```python
from build123d import *
from OCP.BRepFilletAPI import BRepFilletAPI_MakeChamfer

# Parameters (mm, degrees)
SKETCH1_W           = 80
SKETCH1_H           = 60
BOSS_EXTRUDE2_DEPTH = 5
SKETCH3_W           = 15
SKETCH3_H           = 30
BOSS_EXTRUDE3_DEPTH = 25
SKETCH5_R           = 4.1
CUT_EXTRUDE2_DEPTH  = 105.403065089
CHAMFER1_SIZE       = 30
CHAMFER1_SIZE_2     = 10
FILLET1_R           = 15
SKETCH6_R           = 1.5
CUT_EXTRUDE3_DEPTH  = 105.403065089
SKETCH8_R           = 2.5
CUT_EXTRUDE5_DEPTH  = 104.07764064


with BuildPart() as part:
    # Sketch1 → Boss-Extrude2 (new body)
    with BuildSketch(Plane(origin=(0, 0, 0), x_dir=(1, 0, 0), z_dir=(0, 1, 0))):
        with Locations((40, 30)):
            Rectangle(SKETCH1_W, SKETCH1_H)
    extrude(amount=BOSS_EXTRUDE2_DEPTH)

    # Sketch3 → Boss-Extrude3 (add)
    with BuildSketch(Plane(origin=(0, 5, 0), x_dir=(1, 0, 0), z_dir=(0, 1, 0))):
        with Locations((72.5, 45)):
            Rectangle(SKETCH3_W, SKETCH3_H)
        with Locations((47.5, 45)):
            Rectangle(SKETCH3_W, SKETCH3_H)
        with Locations((22.5, 45)):
            Rectangle(SKETCH3_W, SKETCH3_H)
    extrude(amount=BOSS_EXTRUDE3_DEPTH)

    # Sketch5 → Cut-Extrude2 (cut, through all)
    with BuildSketch(Plane(origin=(80, 0, 0), x_dir=(0, 0, -1), z_dir=(1, 0, 0))):
        with Locations((45, 15)):
            Circle(SKETCH5_R)
    extrude(amount=-CUT_EXTRUDE2_DEPTH, mode=Mode.SUBTRACT)

    # Chamfer1
    chamfer1_edges_1 = [part.edges().sort_by_distance(p)[0] for p in [
        (72.5, 5, -30),
    ]]
    chamfer1_side_1 = [part.faces().sort_by_distance(p)[0] for p in [
        (72.5, 5, -29.8),
    ]]
    chamfer1_edges_2 = [part.edges().sort_by_distance(p)[0] for p in [
        (47.5, 5, -30),
    ]]
    chamfer1_side_2 = [part.faces().sort_by_distance(p)[0] for p in [
        (47.5, 5, -29.8),
    ]]
    chamfer1_edges_3 = [part.edges().sort_by_distance(p)[0] for p in [
        (22.5, 5, -30),
    ]]
    chamfer1_side_3 = [part.faces().sort_by_distance(p)[0] for p in [
        (22.5, 5, -29.8),
    ]]
    chamfer1 = BRepFilletAPI_MakeChamfer(part.part.solid().wrapped)
    for e in chamfer1_edges_1:
        chamfer1.Add(CHAMFER1_SIZE - 0.0001, CHAMFER1_SIZE_2 - 0.0001, e.wrapped, chamfer1_side_1[0].wrapped)
    for e in chamfer1_edges_2:
        chamfer1.Add(CHAMFER1_SIZE - 0.0001, CHAMFER1_SIZE_2 - 0.0001, e.wrapped, chamfer1_side_2[0].wrapped)
    for e in chamfer1_edges_3:
        chamfer1.Add(CHAMFER1_SIZE - 0.0001, CHAMFER1_SIZE_2 - 0.0001, e.wrapped, chamfer1_side_3[0].wrapped)
    add(Compound.cast(chamfer1.Shape()), mode=Mode.REPLACE)  # a hair under: the kernel refuses the full size

    # Fillet1
    fillet1_edges = [part.edges().sort_by_distance(p)[0] for p in [
        (72.5, 30, -60),
        (47.5, 30, -60),
        (72.5, 30, -30),
        (47.5, 30, -30),
        (22.5, 30, -60),
        (22.5, 30, -30),
    ]]
    fillet(fillet1_edges, radius=FILLET1_R - 0.0001)  # a hair under: the kernel refuses the full size

    # Sketch6 → Cut-Extrude3 (cut, through all)
    with BuildSketch(Plane.XZ):
        with Locations(Location((72.5, -7.5, 0), (0, 0, 270))):
            Circle(SKETCH6_R)
        with Locations(Location((47.5, -7.5, 0), (0, 0, 270))):
            Circle(SKETCH6_R)
        with Locations(Location((22.5, -7.5, 0), (0, 0, 270))):
            Circle(SKETCH6_R)
    extrude(amount=-CUT_EXTRUDE3_DEPTH, mode=Mode.SUBTRACT)

    # Sketch8 → Cut-Extrude5 (cut, through all)
    with BuildSketch(Plane(origin=(0, 5, 0), x_dir=(1, 0, 0), z_dir=(0, 1, 0))):
        with Locations(Location((22.5, 7.5, 0), (0, 0, 270))):
            Circle(SKETCH8_R)
        with Locations(Location((47.5, 7.5, 0), (0, 0, 270))):
            Circle(SKETCH8_R)
        with Locations(Location((72.5, 7.5, 0), (0, 0, 270))):
            Circle(SKETCH8_R)
    extrude(amount=CUT_EXTRUDE5_DEPTH, mode=Mode.SUBTRACT)


solid = part.part
```
Build history of the part. All positions in model axes, mm. A direction names the side the tool comes from. Give positions to 0.01 mm unless a question says otherwise; leave off trailing zeros. Order: outer loops, then holes, each group sorted by start corner. A loop starts at its lowest first (then second) coordinate and runs counter-clockwise, first axis right, second up. Notation, with made-up numbers: M 33.25,-15 L 39.25,-15 A19 cw 39.25,3 Z; hole C 27,17 d2. An arc over 180 degrees is marked long. Write item = value, one per line. Start each with the question number.
(1) Two-plate mould, pull along Z, no slides. Class faces 1 (the cylindrical face through (22.6, 25.72, -55.49)), 2 (the flat face through (55, 15, -36)), 3 (the cylindrical face through (47.605, 15.18, -40.904)): released by +Z, released by -Z, zero draft, split by the parting line, or undercut.
(2) Probe L1, parallel to X at y = 24, z = -42.5; L2, parallel to X at y = 3.35, z = -7.5; L3, parallel to X at y = 6.7, z = -7.5. List the from-to ranges inside material, lowest first. Write a range as [from, to].
(3) Slice it at C-C on y = 17. Write the cut outline in (x, z).
(4) Pin check, flat tips, straight feed: pin 1 Ø2.5 at (x, z) = (73, -8.5) entering from +Y; pin 2 Ø9.5 at (y, z) = (15, -45) entering from +X; pin 3 Ø1 at (x, z) = (42.5, -39.5) entering from +Y; pin 4 Ø7.5 at (y, z) = (13.5, -37) entering from -X. Stop position of each tip, or through.
(5) Slice it at D-D on z = -16. Write the cut outline in (x, y), plus the area to 3 significant figures.
(6) Slice it at A-A on y = 27.5. Write the cut outline in (x, z).
(7) Slice it at B-B on x = 72.5. State how many separate pieces and enclosed holes the cut face has, plus the area to 3 significant figures.
(8) Which spindle directions (+Z, -Z, +X, -X, +Y, -Y) get a long thin tool onto all of the face, cutting with end or side? Do faces 4 (the flat face through (31, 5, -30)), 5 (the flat face through (39, 0, -30)), 6 (the flat face through (21, 5, -6)), 7 (the flat face through (15, 15, -36)). Say none if no direction does.
Responses:
q1.face_1 = released by -Z
q1.face_2 = zero draft
q1.face_3 = undercut
q2.L1 = [15, 30], [40, 55], [65, 80]
q2.L2 = [0, 21], [24, 46], [49, 71], [74, 80]
q2.L3 = [15, 20], [25, 30], [40, 45], [50, 55], [65, 70], [75, 80]
q3.outline = M 15,-59.87 L 30,-59.87 L 30,-48.58 L 15,-48.58 Z; M 15,-41.42 L 30,-41.42 L 30,-30.13 L 15,-30.13 Z; M 40,-59.87 L 55,-59.87 L 55,-48.58 L 40,-48.58 Z; M 40,-41.42 L 55,-41.42 L 55,-30.13 L 40,-30.13 Z; M 65,-59.87 L 80,-59.87 L 80,-48.58 L 65,-48.58 Z; M 65,-41.42 L 80,-41.42 L 80,-30.13 L 65,-30.13 Z
q4.pin_1 = 5
q4.pin_2 = 80
q4.pin_3 = 29.14
q4.pin_4 = 15
q5.outline = M 0,0 L 80,0 L 80,10.33 L 65,10.33 L 65,5 L 55,5 L 55,10.33 L 40,10.33 L 40,5 L 30,5 L 30,10.33 L 15,10.33 L 15,5 L 0,5 Z
q5.area = 640 mm2
q6.outline = M 15,-53.29 L 30,-53.29 L 30,-36.71 L 15,-36.71 Z; M 40,-53.29 L 55,-53.29 L 55,-36.71 L 40,-36.71 Z; M 65,-53.29 L 80,-53.29 L 80,-36.71 L 65,-36.71 Z
q7.separate_pieces = 2
q7.enclosed_holes = 1
q7.area = 1,020 mm2
q8.face_4 = +Z, -Z, +Y
q8.face_5 = +Z, -Z, +X, -X, -Y
q8.face_6 = +Y
q8.face_7 = +Z, -Z, -X, +Y
